```python
from build123d import *

# Parameters (mm, degrees)
F1_DEPTH = 25
F2_R     = 1.5
F3_DEPTH = 3
F4_R     = 1.5
F5_DEPTH = 3
F7_DEPTH = 3
F8_R     = 6
F9_DEPTH = 3


with BuildPart() as f1:
    # F0 (on Right) → F1 (new body)
    with BuildSketch(Plane.YZ):
        Polygon((0, -3), (0, 0), (-7, 0), (-7, 35), (58, 35), (58, 27), (61, 27), (61, 38), (-10, 38), (-10, -3), align=None)
    extrude(amount=F1_DEPTH)

    # F2 (on face) → F3 (cut)
    with BuildSketch(Plane(origin=(0, 0, -3), x_dir=(1, 0, 0), z_dir=(0, 0, -1))):
        with Locations((20.5, 4.5)):
            Circle(F2_R)
        with Locations((4.5, 4.5)):
            Circle(F2_R)
    extrude(amount=-F3_DEPTH, mode=Mode.SUBTRACT)

    # F4 (on face) → F5 (cut)
    with BuildSketch(Plane(origin=(0, 61, 0), x_dir=(-1, 0, 0), z_dir=(0, 1, 0))):
        with Locations((-20.5, 31.5)):
            Circle(F4_R)
        with Locations((-4.5, 31.5)):
            Circle(F4_R)
    extrude(amount=-F5_DEPTH, mode=Mode.SUBTRACT)

    # F6 (on face) → F7 (join)
    with BuildSketch(Plane.XY.offset(38)):
        with BuildLine():
            Line((0, 16.0444763524), (0, 20.2350013331))
            Line((0, 20.2350013331), (-15, 20.2350013331))
            Line((-15, 20.2350013331), (-15, 0.2350013331))
            Line((-15, 0.2350013331), (0, 0.2350013331))
            Line((0, 0.2350013331), (0, 4.4255263137))
            ThreePointArc((0, 4.4255263137), (-4.5, 10.2350013331), (0, 16.0444763524))
        make_face()
        with BuildLine():
            Line((0, 13.9431005766), (0, 16.0444763524))
            ThreePointArc((0, 16.0444763524), (-4.5, 10.2350013331), (0, 4.4255263137))
            Line((0, 4.4255263137), (0, 6.5269020895))
            ThreePointArc((0, 6.5269020895), (-2.5, 10.2350013331), (0, 13.9431005766))
        make_face()
        with BuildLine():
            Line((40, 20.2350013331), (25, 20.2350013331))
            Line((25, 20.2350013331), (25, 16.0444763524))
            ThreePointArc((25, 16.0444763524), (28.2434164903, 13.9092359472), (29.5, 10.2350013331))
            ThreePointArc((29.5, 10.2350013331), (28.2434164903, 6.5607667189), (25, 4.4255263137))
            Line((25, 4.4255263137), (25, 0.2350013331))
            Line((25, 0.2350013331), (40, 0.2350013331))
            Line((40, 0.2350013331), (40, 20.2350013331))
        make_face()
        with BuildLine():
            Line((25, 13.9431005766), (25, 16.0444763524))
            ThreePointArc((25, 16.0444763524), (17.5, 10.2350013331), (25, 4.4255263137))
            Line((25, 4.4255263137), (25, 6.5269020895))
            ThreePointArc((25, 6.5269020895), (19.5, 10.2350013331), (25, 13.9431005766))
        make_face()
        with BuildLine():
            Line((25, 6.5269020895), (25, 13.9431005766))
            ThreePointArc((25, 13.9431005766), (19.5, 10.2350013331), (25, 6.5269020895))
        make_face()
    extrude(amount=-F7_DEPTH)

    # F8 (on face) → F9 (cut)
    with BuildSketch(Plane.XY.offset(38)):
        with Locations((1.5, 10.2350013331)):
            Circle(F8_R)
        with BuildLine():
            ThreePointArc((0, 6.5269020895), (-2.5, 10.2350013331), (0, 13.9431005766))
            Line((0, 13.9431005766), (0, 6.5269020895))
        make_face(mode=Mode.SUBTRACT)
        with BuildLine():
            Line((25, 4.4255263137), (25, 16.0444763524))
            ThreePointArc((25, 16.0444763524), (17.5, 10.2350013331), (25, 4.4255263137))
        make_face()
        with BuildLine():
            ThreePointArc((25, 4.4255263137), (28.2434164903, 6.5607667189), (29.5, 10.2350013331))
            ThreePointArc((29.5, 10.2350013331), (28.2434164903, 13.9092359472), (25, 16.0444763524))
            Line((25, 16.0444763524), (25, 4.4255263137))
        make_face()
    extrude(amount=-F9_DEPTH, mode=Mode.SUBTRACT)


solid = f1.part
```
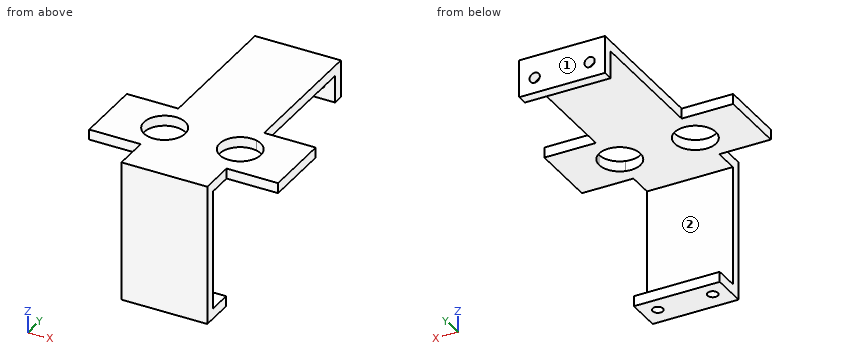
Here's how the part is built. I have some questions about the finished solid (model axes, mm). Face numbers are marked on the shaded views. A direction names the side the tool comes from. Coordinates: 2 decimals unless noted, no trailing zeros. Order: outer loops, then holes, each group sorted by start corner. A loop starts at its lowest first (then second) coordinate and runs counter-clockwise, first axis right, second up. Notation, with made-up numbers: (34.25, -25) -> (86.25, -25) arc R20 cw to (86.25, -20) -> close; hole circle Ø4 at (-14, 68.25). An arc over 180 degrees is marked (long way). Return JSON: item names as keys, results as strings.
1) If we section it at A-A on z = 31.5: List the corners of the cut face in (x, y) for me, plus the area to 3 significant figures.
Conclusion:
{"outline": "(0, -10) -> (25, -10) -> (25, -7) -> (0, -7) -> close; (0, 58) -> (3, 58) -> (3, 61) -> (0, 61) -> close; (6, 58) -> (19, 58) -> (19, 61) -> (6, 61) -> close; (22, 58) -> (25, 58) -> (25, 61) -> (22, 61) -> close", "area": "132 mm²"}
2) On a 3-axis mill with a long thin cutter (end or side, diameter ignored), from which of +Z, -Z, +X, -X, +Y, -Y can I reach the whole of each face in a straight line? I mean the marked faces 1 and 2. Say none if no direction works.
Conclusion:
{"face 1": "+Z, -Z, +X, -X, +Y", "face 2": "+X, -X"}
3) If we section it at C-C on x = 23.5: List the corners of the cut face in (y, z) for me (3 decimals).
Conclusion:
{"outline": "(-10, -3) -> (0, -3) -> (0, 0) -> (-7, 0) -> (-7, 35) -> (4.235, 35) -> (4.235, 38) -> (-10, 38) -> close; (16.235, 35) -> (58, 35) -> (58, 27) -> (61, 27) -> (61, 38) -> (16.235, 38) -> close"}
4) If we section it at D-D on x = 14.5: List the corners of the cut face in (y, z) for me.
Conclusion:
{"outline": "(-10, -3) -> (0, -3) -> (0, 0) -> (-7, 0) -> (-7, 35) -> (58, 35) -> (58, 27) -> (61, 27) -> (61, 38) -> (-10, 38) -> close"}
5) I'm going to push flat-ended pins straight in: P1, Ø8, axis at x = 3.5, y = 43.5, coming from the -Z side; P2, Ø1.5, axis at x = -9.5, z = 36.5, coming from the -Y side (3 decimals); P3, Ø8, axis at y = -4.5, z = 24, coming from the +X side. Where does each tip first touch, or does it pass through?
Conclusion:
{"P1": "stops at z = 35", "P2": "stops at y = 0.235", "P3": "stops at x = 25"}
6) If we section it at B-B on y = -4.5: List the corners of the cut face in (x, z) for me.
Conclusion:
{"outline": "(0, -3) -> (3, -3) -> (3, 0) -> (0, 0) -> close; (0, 35) -> (25, 35) -> (25, 38) -> (0, 38) -> close; (6, -3) -> (19, -3) -> (19, 0) -> (6, 0) -> close; (22, -3) -> (25, -3) -> (25, 0) -> (22, 0) -> close"}
7) If I drill on probe 1 along X at (y, z) = (-4.5, -2.35); probe 2 along Y at (x, z) = (21.5, 33); probe 3 along Y at (x, z) = (4.5, -1.5), over which ranges is the centre line in solid material (lowest first)?
Conclusion:
{"probe 1": "x = 0 to 3, 6 to 19, 22 to 25", "probe 2": "y = -10 to -7, 58 to 61", "probe 3": "y = -10 to -6, -3 to 0"}
